```python
from build123d import *

# Parameters (mm, degrees)
SKETCH4_R                = 16
SKETCH4_R_2              = 13.25
BOSS_EXTRUDE3_DEPTH      = 150
BOSS_EXTRUDE4_DEPTH      = 10
BOSS_EXTRUDE4_DEPTH_BACK = 4
SKETCH6_R                = 9.7
SKETCH6_R_2              = 7.5
SKETCH7_R                = 7.5
CUT_EXTRUDE1_DEPTH       = 20
CUT_EXTRUDE2_START       = -150
SKETCH8_R                = 13.25
CUT_EXTRUDE2_DEPTH       = 150
SKETCH11_R               = 1.6
CUT_EXTRUDE5_DEPTH       = 13
CUT_EXTRUDE7_DEPTH       = 42.3
SKETCH15_W               = 60
SKETCH15_H               = 10
SKETCH15_R               = 1.6
BOSS_EXTRUDE5_DEPTH      = 5
SKETCH16_R               = 13.25
CUT_EXTRUDE8_DEPTH       = 150
FILLET2_R                = 3
FILLET3_R                = 5
CUT_EXTRUDE10_START      = 4
SKETCH20_R               = 4.747407389
SKETCH20_W               = 2.1
SKETCH20_H               = 3
CUT_EXTRUDE10_DEPTH      = 6
BOSS_EXTRUDE6_START      = -0.5
BOSS_EXTRUDE6_DEPTH      = 5
FILLET4_R                = 0.5
CUT_EXTRUDE11_DEPTH      = 4
CUT_EXTRUDE12_DEPTH      = 3


# Some blends are built 0.0001 mm under size
with BuildPart() as part:
    # Sketch4 → Boss-Extrude3 (new body)
    with BuildSketch(Plane.XY):
        Circle(SKETCH4_R)
        Circle(SKETCH4_R_2, mode=Mode.SUBTRACT)
    extrude(amount=BOSS_EXTRUDE3_DEPTH)

    # Sketch6 → Boss-Extrude4 (add, two sides: drawn at the far end of the back side and taken through both)
    with BuildSketch(Plane(origin=(0, 16, 150), x_dir=(1, 0, 0), z_dir=(0, 1, 0)).offset(-BOSS_EXTRUDE4_DEPTH_BACK)):
        with Locations(Location((0, 80, 0), (0, 0, 180))):
            Circle(SKETCH6_R)
        with Locations(Location((0, 80, 0), (0, 0, 180))):
            Circle(SKETCH6_R_2, mode=Mode.SUBTRACT)
    extrude(amount=BOSS_EXTRUDE4_DEPTH + BOSS_EXTRUDE4_DEPTH_BACK)

    # Sketch7 → Cut-Extrude1 (cut)
    with BuildSketch(Plane(origin=(0, 26, 0), x_dir=(1, 0, 0), z_dir=(0, 1, 0))):
        with Locations(Location((0, -70, 0), (0, 0, 180))):
            Circle(SKETCH7_R)
    extrude(amount=-CUT_EXTRUDE1_DEPTH, mode=Mode.SUBTRACT)

    # Sketch8 → Cut-Extrude2 (cut)
    with BuildSketch(Plane.XY.offset(150).offset(CUT_EXTRUDE2_START)):
        Circle(SKETCH8_R)
    extrude(amount=CUT_EXTRUDE2_DEPTH, mode=Mode.SUBTRACT)

    # Sketch11 → Cut-Extrude5 (cut)
    with BuildSketch(Plane(origin=(0, 16, 150), x_dir=(1, 0, 0), z_dir=(0, 1, 0))):
        with Locations(Location((0, 12, 0), (0, 0, 180))):
            Circle(SKETCH11_R)
    extrude(amount=-CUT_EXTRUDE5_DEPTH, mode=Mode.SUBTRACT)

    # Sketch14 → Cut-Extrude7 (cut)
    with BuildSketch(Plane.ZY.offset(16)):
        Polygon((150, 16), (130, -16), (150, -16), align=None)
    extrude(amount=-CUT_EXTRUDE7_DEPTH, mode=Mode.SUBTRACT)

    # Sketch15 → Boss-Extrude5 (add)
    with BuildSketch(Plane(origin=(0, -16, 150), x_dir=(-1, 0, 0), z_dir=(0, -1, 0))):
        with Locations((0, 135)):
            Rectangle(SKETCH15_W, SKETCH15_H)
        with Locations(Location((-25, 135, 0), (0, 0, 180))):
            Circle(SKETCH15_R, mode=Mode.SUBTRACT)
        with Locations(Location((25, 135, 0), (0, 0, 180))):
            Circle(SKETCH15_R, mode=Mode.SUBTRACT)
    extrude(amount=-BOSS_EXTRUDE5_DEPTH)

    # Sketch16 → Cut-Extrude8 (cut)
    with BuildSketch(Plane(origin=(0, 0, 0), x_dir=(-1, 0, 0), z_dir=(0, 0, -1))):
        with Locations(Location((0, 0, 0), (0, 0, 270))):
            Circle(SKETCH16_R)
    extrude(amount=-CUT_EXTRUDE8_DEPTH, mode=Mode.SUBTRACT)

    # Fillet2
    # the kernel refuses this fillet: 3 mm, written as the material it takes off along each edge
    with BuildSketch(Plane(origin=(0, 26, 70), x_dir=(-1, 0, 0), z_dir=(0, 0, -1))) as fillet2_piece_1:
        with BuildLine():
            CenterArc((10.5, -2.891366459), FILLET2_R, 105.466009953, 74.533990047)
            Line((7.5, -2.891366459), (7.44, -2.891366459))
            Line((7.44, -2.891366459), (7.44, 0))
            Line((7.44, 0), (7.5, 0.06))
            ThreePointArc((7.5, 0.06), (8.6, 0.06), (9.684, 0.057827329))
            Line((9.684, 0.057827329), (9.7, 0))
        make_face()
    revolve(axis=Axis((0, 26, 70), (0, 1, 0)), mode=Mode.SUBTRACT)

    # Fillet3
    fillet3_edges = [part.edges().sort_by_distance(p)[0] for p in [
        (11.618950039, -11, 15),
        (-11.618950039, -11, 15),
    ]]
    fillet(fillet3_edges, radius=FILLET3_R)

    # Sketch20 → Cut-Extrude10 (cut)
    with BuildSketch(Plane(origin=(0, 16, 150), x_dir=(1, 0, 0), z_dir=(0, 1, 0)).offset(CUT_EXTRUDE10_START)):
        with Locations((0, 80)):
            Circle(SKETCH20_R)
        with Locations((0, 88.2)):
            Rectangle(SKETCH20_W, SKETCH20_H)
        with Locations((0, 71.8)):
            Rectangle(SKETCH20_W, SKETCH20_H)
    extrude(amount=CUT_EXTRUDE10_DEPTH, mode=Mode.SUBTRACT)

    # Sketch21 → Boss-Extrude6 (add)
    with BuildSketch(Plane(origin=(0, 0, 0), x_dir=(-1, 0, 0), z_dir=(0, 0, -1)).offset(BOSS_EXTRUDE6_START)):
        with BuildLine():
            Line((-17.5, -5.75), (-17.5, -1.127899498))
            Line((-17.5, -1.127899498), (-20.098498502, -2.315784528))
            ThreePointArc((-20.098498502, -2.315784528), (-23.184215472, -10.598498502), (-14.901501498, -13.684215472))
            Line((-14.901501498, -13.684215472), (-10.796967628, -11.807857132))
            ThreePointArc((-10.796967628, -11.807857132), (-12.472856829, -10.021369294), (-13.856406461, -8))
            Line((-13.856406461, -8), (-15.25, -8))
            ThreePointArc((-15.25, -8), (-19.090990258, -9.590990258), (-17.5, -5.75))
        make_face()
        with BuildLine():
            ThreePointArc((-13.856406461, -8), (-15.396484426, -4.352960754), (-15.993964631, -0.439426187))
            Line((-15.993964631, -0.439426187), (-17.5, -1.127899498))
            Line((-17.5, -1.127899498), (-17.5, -5.75))
            ThreePointArc((-17.5, -5.75), (-15.909009742, -6.409009742), (-15.25, -8))
            Line((-15.25, -8), (-13.856406461, -8))
        make_face()
        with BuildLine():
            Line((20.098498502, -2.315784528), (17.5, -1.127899498))
            Line((17.5, -1.127899498), (17.5, -5.75))
            ThreePointArc((17.5, -5.75), (19.090990258, -6.409009742), (19.75, -8))
            ThreePointArc((19.75, -8), (17.5, -10.25), (15.25, -8))
            Line((15.25, -8), (13.856406461, -8))
            ThreePointArc((13.856406461, -8), (12.472856829, -10.021369294), (10.796967628, -11.807857132))
            Line((10.796967628, -11.807857132), (14.901501498, -13.684215472))
            ThreePointArc((14.901501498, -13.684215472), (23.184215472, -10.598498502), (20.098498502, -2.315784528))
        make_face()
        with BuildLine():
            Line((17.5, -5.75), (17.5, -1.127899498))
            Line((17.5, -1.127899498), (15.993964631, -0.439426187))
            ThreePointArc((15.993964631, -0.439426187), (15.396484426, -4.352960754), (13.856406461, -8))
            Line((13.856406461, -8), (15.25, -8))
            ThreePointArc((15.25, -8), (15.909009742, -6.409009742), (17.5, -5.75))
        make_face()
    extrude(amount=-BOSS_EXTRUDE6_DEPTH)

    # Fillet4
    fillet4_edges = [part.edges().sort_by_distance(p)[0] for p in [
        (14.551591609, -6.652156164, 0.5),
        (-14.551591609, -6.652156164, 0.5),
    ]]
    fillet(fillet4_edges, radius=FILLET4_R - 0.0001)  # a hair under: the kernel refuses the full size

    # Sketch22 → Cut-Extrude11 (cut)
    with BuildSketch(Plane.XY.offset(5.5)):
        Polygon((15.993964631, -0.439426187), (10.796967628, -11.807857132), (12.161179341, -12.431496772), (17.358176345, -1.063065827), align=None)
        Polygon((-15.993964631, -0.439426187), (-10.796967628, -11.807857132), (-12.161179341, -12.431496772), (-17.358176345, -1.063065827), align=None)
    extrude(amount=CUT_EXTRUDE11_DEPTH, mode=Mode.SUBTRACT)

    # Sketch23 → Cut-Extrude12 (cut)
    with BuildSketch(Plane.XY.offset(5.5)):
        Polygon((-19.126954006, -4.441038113), (-21.395628408, -7.629502556), (-19.768674403, -11.188464443), (-15.873045994, -11.558961887), (-13.604371592, -8.370497444), (-15.231325597, -4.811535557), align=None)
        Polygon((19.175049478, -4.335829267), (15.1642598, -4.717279233), (13.489210323, -8.381449966), (15.824950522, -11.664170733), (19.8357402, -11.282720767), (21.510789677, -7.618550034), align=None)
    extrude(amount=-CUT_EXTRUDE12_DEPTH, mode=Mode.SUBTRACT)


solid = part.part
```
Design review of the part built by this model. Coordinates are the model's own, in mm. A direction names the side the tool comes from. Give positions to 0.01 mm unless a question says otherwise; leave off trailing zeros. Write each loop counter-clockwise with the first axis right and the second up, starting at its lowest first coordinate (ties: lowest second). Pieces come first, ordered by that corner, then holes. Notation, with made-up numbers: (46.25, 17.5) - (98.25, 17.5) arc R21 cw to (98.25, 50.5) - close; hole circle Ø7 at (64, -40). An arc over 180 degrees is marked (long way). Return JSON: item names as keys, results as strings. Group by question number.
(1) Machinability: for faces 5 (the flat face through (-12.821, -12.733, 2.712)), 6 (the flat face through (-14, -7, 9.5)), 7 (the flat face through (-17.85, -11.37, 4.02)), 8 (the flat face through (20, -9, 0.5)), 9 (the flat face through (19, -13, 10)), which of the approach directions +Z, -Z, +X, -X, +Y, -Y give a long, thin tool a straight path to every point of the face, cutting with its end or side? Answer none if there is none.
(2) We need section A-A, the plane z = 15. Give the boundary of the cut face in (x, y).
(3) Insertion check: pin 1 (5.5 mm diameter, centred on x = -13, y = -8.5, fed in from -Z); pin 2 (4 mm diameter, centred on x = 19, y = -6.5, fed in from +Z); pin 3 (8 mm diameter, centred on x = 26.5, z = 13, fed in from +Y); pin 4 (12 mm diameter, centred on y = -5.5, z = 115.5, fed in from +X). Each pin has a flat end and moves straight along its axis. Give the tip position at first contact, or say it passes through.
(4) We need section B-B, the plane z = 70. Give the boundary of the cut face in (x, y), then the cut area to 3 significant figures.
(5) Mouldability with a two-part tool opening along X and no side actions: class faces 1 (the flat face through (-14.755, -9.987, 4.021)), 2 (the flat face through (-16, -10, 2.5)), 3 (the cylindrical face through (16.155, -9.04, 14.93)), 4 (the flat face through (27, -11, 15)) as +X half, -X half, draft (parallel to the pull), parting line (faces both ways), or undercut.
(6) We need section C-C, the plane z = 138. Give the boundary of the cut face in (x, y).
(7) We need section D-D, the plane z = 45. Give the boundary of the cut face in (x, y).
(8) To check wall thickness, follow probe 1 along Y at (x, z) = (0, 101); probe 2 along Z at (x, y) = (16.5, -11.5); probe 3 along X at (y, z) = (-8, 1). State the ranges of each line that lie inside material, in increasing order.
Reported:
{
 "1": {"face 5": "-Z, -Y", "face 6": "-X, -Y", "face 7": "none", "face 8": "-Z, +X, -Y", "face 9": "+X, -Y"},
 "2": {"outline": "(-30, -16) - (-26.6, -16) - (-26.6, -11) - (-30, -11) - close; (-23.4, -16) - (23.4, -16) - (23.4, -11) - (20.12, -11) arc R5 cw to (15.33, -4.57) arc R16 ccw (long way) to (-15.33, -4.57) arc R5 cw to (-20.12, -11) - (-23.4, -11) - close; (26.6, -16) - (30, -16) - (30, -11) - (26.6, -11) - close; hole circle Ø26.5 at (0, 0)"},
 "3": {"pin 1": "stops at z = 0", "pin 2": "stops at z = 5.5", "pin 3": "stops at y = -11", "pin 4": "stops at x = 16"},
 "4": {"outline": "(-9.7, 12.72) arc R16 ccw (long way) to (9.7, 12.72) - (9.7, 26) arc R3 ccw to (7.5, 23.11) - (7.5, 10.92) arc R13.25 cw (long way) to (-7.5, 10.92) - (-7.5, 23.11) arc R3 ccw to (-9.7, 26) - close", "area": "261 mm2"},
 "5": {"face 1": "undercut", "face 2": "undercut", "face 3": "+X half", "face 4": "draft"},
 "6": {"outline": "(-15.68, -3.2) - (-12.86, -3.2) arc R13.25 cw to (-1.6, 13.15) - (-1.6, 15.92) arc R16 ccw to start; (1.6, 13.15) arc R13.25 cw to (12.86, -3.2) - (15.68, -3.2) arc R16 ccw to (1.6, 15.92) - close"},
 "7": {"outline": "circle Ø32 at (0, 0); hole circle Ø26.5 at (0, 0)"},
 "8": {"probe 1": "y = -16 to -13.25, 13.25 to 16", "probe 2": "z = 0.5 to 2.5, 10 to 20", "probe 3": "x = -23.75 to -19.75, -15.25 to -10.56, 10.56 to 15.25, 19.75 to 23.75"}
}
